```python
from build123d import *

# Parameters (mm, degrees)
SKETCH2_R           = 3.25
SKETCH2_R_2         = 4
BOSS_EXTRUDE1_DEPTH = 5


with BuildPart() as part:
    # Sketch2 → Boss-Extrude1 (new body)
    with BuildSketch(Plane(origin=(0, 0, 0), x_dir=(1, 0, 0), z_dir=(0, 1, 0))):
        with BuildLine():
            ThreePointArc((74.0754883, 100.6287171), (72.919899742, 100.600095739), (72.5093633, 101.680680732))
            ThreePointArc((72.5093633, 101.680680732), (77.933093033, 110.354945232), (87.35286635, 114.345882401))
            ThreePointArc((87.35286635, 114.345882401), (87.962324772, 113.982635249), (87.79926183, 113.292129247))
            ThreePointArc((87.79926183, 113.292129247), (88.97179336, 110.122737844), (90.12915105, 113.29770166))
            ThreePointArc((90.12915105, 113.29770166), (89.96425768, 113.984397711), (90.570273688, 114.34700754))
            ThreePointArc((90.570273688, 114.34700754), (100.167880321, 110.211447196), (105.532711055, 101.242862936))
            ThreePointArc((105.532711055, 101.242862936), (105.075581876, 100.162342656), (103.906399753, 100.259832785))
            ThreePointArc((103.906399753, 100.259832785), (97.726174894, 97.422732696), (103.906399753, 94.585632606))
            ThreePointArc((103.906399753, 94.585632606), (105.075581876, 94.683122735), (105.532711055, 93.602602455))
            ThreePointArc((105.532711055, 93.602602455), (100.172351893, 84.637935793), (90.582110249, 80.49958299))
            ThreePointArc((90.582110249, 80.49958299), (89.972651827, 80.862830142), (90.135714769, 81.553336144))
            ThreePointArc((90.135714769, 81.553336144), (88.963183239, 84.722727547), (87.805825549, 81.547763731))
            ThreePointArc((87.805825549, 81.547763731), (87.97071892, 80.86106768), (87.364702911, 80.498457852))
            ThreePointArc((87.364702911, 80.498457852), (77.937616147, 84.486662184), (72.5093633, 93.164784659))
            ThreePointArc((72.5093633, 93.164784659), (72.919899742, 94.245369652), (74.0754883, 94.216748291))
            ThreePointArc((74.0754883, 94.216748291), (80.4674883, 97.422732696), (74.0754883, 100.6287171))
        make_face()
        with Locations(Location((80.9674883, 89.422732696, 0), (0, 0, 270))):
            Circle(SKETCH2_R, mode=Mode.SUBTRACT)
        with Locations(Location((88.9674883, 97.422732696, 0), (0, 0, 270))):
            Circle(SKETCH2_R_2, mode=Mode.SUBTRACT)
        with Locations(Location((80.9674883, 105.422732696, 0), (0, 0, 270))):
            Circle(SKETCH2_R, mode=Mode.SUBTRACT)
        with Locations(Location((96.9674883, 105.422732696, 0), (0, 0, 270))):
            Circle(SKETCH2_R, mode=Mode.SUBTRACT)
        with Locations(Location((96.9674883, 89.422732696, 0), (0, 0, 270))):
            Circle(SKETCH2_R, mode=Mode.SUBTRACT)
    extrude(amount=BOSS_EXTRUDE1_DEPTH)


solid = part.part
```
Geometry check sheet. Reference: the model listing, model coordinates, mm. A direction names the side the tool comes from. Round coordinates to 2 decimals unless told otherwise and drop trailing zeros. Loops run counter-clockwise (first coordinate to the right, second up) from the corner with the lowest first, then second, coordinate; pieces in that order, holes last. Notation, with made-up numbers: M -40,19.5 L 13,19.5 A29 ccw 13,40.5 Z; hole C -8,-0.5 d6. An arc over 180 degrees is marked long. Return JSON: item names as keys, results as strings. Group by question number.
(1) Mould release check, pull along Z, two halves, no side actions. Record for faces 1 (the face through (100.284, 2.465, -84.736)), 2 (the face through (93, 5, -101)), 3 (the face through (94.99, 2.46, -92)): pulls with the +Z half, pulls with the -Z half, needs draft (parallel to the pull), parting line crosses it, or undercut.
(2) Set-up check for faces 4 (the face through (93, 0, -101)), 5 (the face through (89.98, 2.46, -80.85)): record each of +Z, -Z, +X, -X, +Y, -Y from which the full face is reachable in a straight line by a thin tool's end or side.
(3) Go/stop test with flat-tipped pins: pin 1 (1.5 mm diameter, centred on x = 99.5, y = 2, fed in from -Z); pin 2 (1.5 mm diameter, centred on y = 3, z = -88, fed in from -X). Record where each tip stops, or that it passes through.
(4) Section check B-B, the plane x = 83. Enter the section's corners in (y, z), and give its area (3 significant figures).
(5) Section check A-A, the plane z = -99.5. Enter the section's corners in (x, y).
(6) Section check C-C, the plane z = -91. Enter the section's corners in (x, y), and give its area (3 significant figures).
(7) Scan lines: line 1 along X through (y, z) = (3.3, -92); line 2 along Z through (x, y) = (95.5, 0.65); line 3 along Z through (x, y) = (83, 1.15). Record each from-to range of solid material in increasing order. Write a range as [from, to].
(8) Section check D-D, the plane x = 77. Enter the section's corners in (y, z), and give its area (3 significant figures).
Data:
{
 "1": {"face 1": "pulls with the +Z half", "face 2": "needs draft", "face 3": "undercut"},
 "2": {"face 4": "+Z, -Z, +X, -X, -Y", "face 5": "+Y, -Y"},
 "3": {"pin 1": "z = -111.33", "pin 2": "x = 74.35"},
 "4": {"outline": "M 0,-113.34 L 5,-113.34 L 5,-107.96 L 0,-107.96 Z; M 0,-102.89 L 5,-102.89 L 5,-91.96 L 0,-91.96 Z; M 0,-86.89 L 5,-86.89 L 5,-81.5 L 0,-81.5 Z", "area": "108 mm²"},
 "5": {"outline": "M 79.89,0 L 85.55,0 L 85.55,5 L 79.89,5 Z; M 92.39,0 L 98.36,0 L 98.36,5 L 92.39,5 Z"},
 "6": {"outline": "M 73.23,0 L 78.13,0 L 78.13,5 L 73.23,5 Z; M 83.81,0 L 94.13,0 L 94.13,5 L 83.81,5 Z; M 99.81,0 L 104.71,0 L 104.71,5 L 99.81,5 Z", "area": "101 mm²"},
 "7": {"line 1": "[72.86, 78.99], [82.95, 94.99], [98.95, 105.08]", "line 2": "[-113.12, -108.32], [-102.52, -92.32], [-86.52, -81.73]", "line 3": "[-113.34, -107.96], [-102.89, -91.96], [-86.89, -81.5]"},
 "8": {"outline": "M 0,-109.5 L 5,-109.5 L 5,-101.39 L 0,-101.39 Z; M 0,-93.46 L 5,-93.46 L 5,-85.35 L 0,-85.35 Z", "area": "81.1 mm²"}
}
